from build123d import *

# Parameters (mm, degrees)
EXTRUDE_1_DEPTH     = 3
SKETCH_2_R          = 2
CUT_EXTRUDE_1_DEPTH = 3


with BuildPart() as part:
    # 草图1 → 凸台-拉伸1 (new body)
    with BuildSketch(Plane.XY):
        Polygon((0, 0), (90, 0), (90, -20), (85, -20), (65, -40), (65, -45), (25, -45), (25, -40), (5, -20), (0, -20), align=None)
    extrude(amount=EXTRUDE_1_DEPTH)

    # 草图2 → 切除-拉伸1 (cut)
    with BuildSketch(Plane.XY.offset(3)):
        with Locations((82, -5)):
            Circle(SKETCH_2_R)
        with Locations((82, -15.5)):
            Circle(SKETCH_2_R)
        with Locations((64, -15.5)):
            Circle(SKETCH_2_R)
        with Locations((64, -5)):
            Circle(SKETCH_2_R)
        with Locations((26, -5)):
            Circle(SKETCH_2_R)
        with Locations((26, -15.5)):
            Circle(SKETCH_2_R)
        with Locations((8, -5)):
            Circle(SKETCH_2_R)
        with Locations((8, -15.5)):
            Circle(SKETCH_2_R)
        with Locations((31, -27)):
            Circle(SKETCH_2_R)
        with Locations((31, -39)):
            Circle(SKETCH_2_R)
        with Locations((59, -27)):
            Circle(SKETCH_2_R)
        with Locations((59, -39)):
            Circle(SKETCH_2_R)
        with BuildLine():
            Line((52.5, -11.5), (52.5, -33.5))
            ThreePointArc((52.5, -33.5), (45, -41), (37.5, -33.5))
            Line((37.5, -33.5), (37.5, -11.5))
            ThreePointArc((37.5, -11.5), (45, -4), (52.5, -11.5))
        make_face()
    extrude(amount=-CUT_EXTRUDE_1_DEPTH, mode=Mode.SUBTRACT)


solid = part.part
Work out the finished part from the listing and answer in its coordinate system (mm). A direction names the side the tool comes from. Coordinates: 2 decimals unless noted, no trailing zeros. Write each loop counter-clockwise with the first axis right and the second up, starting at its lowest first coordinate (ties: lowest second). Pieces come first, ordered by that corner, then holes.
1. For faces 1 (the cylindrical face through (45, -4, 2)), 2 (the flat face through (3, -20, 1)), 3 (the flat face through (56, -17, 3)), determine the directions among +Z, -Z, +X, -X, +Y, -Y from which every point of the face is accessible in a straight line to the end or side of a thin tool.
Results list:
face 1: +Z, -Z
face 2: +Z, -Z, -X, -Y
face 3: +Z, +X, -X, +Y, -Y
2. Consider line 1 along Y through (x, z) = (31, 1.55); line 2 along Y through (x, z) = (64, 2.25); line 3 along X through (y, z) = (-17, 1.1). Determine where each line is inside the solid, lowest interval first.
Results list:
line 1: y = -45 to -41, -37 to -29, -25 to 0
line 2: y = -45 to -17.5, -13.5 to -7, -3 to 0
line 3: x = 0 to 6.68, 9.32 to 24.68, 27.32 to 37.5, 52.5 to 62.68, 65.32 to 80.68, 83.32 to 90
3. The part is cut by section B-B, the plane z = 2.15. State how many separate pieces and enclosed holes the cut face has, and give its area (3 significant figures).
Results list:
separate pieces: 1
enclosed holes: 13
area: 2,540 mm2
4. The part is cut by section C-C, the plane x = 59. Write down the section's boundary in (y, z), and give its area (3 significant figures).
Results list:
outline: (-45, 0) - (-41, 0) - (-41, 3) - (-45, 3) - close; (-37, 0) - (-29, 0) - (-29, 3) - (-37, 3) - close; (-25, 0) - (0, 0) - (0, 3) - (-25, 3) - close
area: 111 mm2
5. The part is cut by section D-D, the plane y = -39. Write down the section's boundary in (x, z).
Results list:
outline: (24, 0) - (29, 0) - (29, 3) - (24, 3) - close; (33, 0) - (39.9, 0) - (39.9, 3) - (33, 3) - close; (50.1, 0) - (57, 0) - (57, 3) - (50.1, 3) - close; (61, 0) - (66, 0) - (66, 3) - (61, 3) - close
6. A flat-ended cylindrical pin translates along its axis: pin 1 (0.9 mm diameter, centred on y = -41.5, z = 1, fed in from +X). Find the tip coordinate at first contact, or state that the pin passes through.
Results list:
pin 1: stops at x = 65
7. For a pull along Y with two mould halves and no side action, classify faces 4 (the cylindrical face through (45, -41, 2)), 5 (the flat face through (88, -20, 1)), 6 (the flat face through (65, -42, 1)) as +Y half, -Y half, draft (parallel to the pull), parting line (faces both ways), or undercut.
Results list:
face 4: undercut
face 5: -Y half
face 6: draft
8. The part is cut by section A-A, the plane x = 45. Write down the section's boundary in (y, z), and give its area (3 significant figures).
Results list:
outline: (-45, 0) - (-41, 0) - (-41, 3) - (-45, 3) - close; (-4, 0) - (0, 0) - (0, 3) - (-4, 3) - close
area: 24.0 mm2
